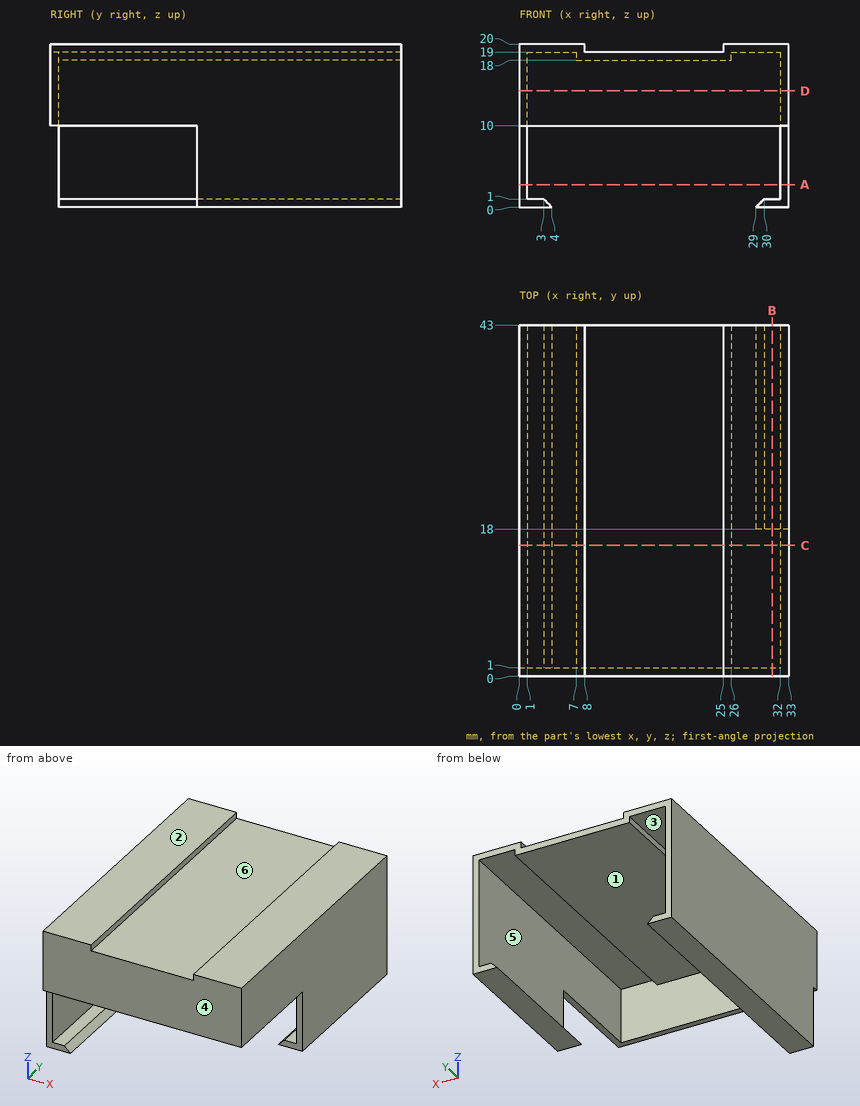
Print and shaded views of the part. All mm, measured from the part's lowest x, y and z. A direction names the side the tool comes from. Coordinates: 2 decimals unless noted, no trailing zeros. Order: outer loops, then holes, each group sorted by start corner. A loop starts at its lowest first (then second) coordinate and runs counter-clockwise, first axis right, second up. Notation, with made-up numbers: M 31,46.5 L 38,46.5 A9 cw 38,57.5 Z; hole C 20.25,22 d1. An arc over 180 degrees is marked long. Write each question's results on one line, items separated by ' | '. Start each with the question number.
Q1. Cut at C-C (y = 16). List the corners of the cut face in (x, z).
Q2. Which spindle directions (+Z, -Z, +X, -X, +Y, -Y) get a long thin tool onto all of the face, cutting with end or side? Do the marked faces 4, 5 and 6. Say none if no direction does.
Q3. Pull direction Z, two halves, no side cores. Call the marked faces 1, 2 and 3: +Z half, -Z half, draft (parallel to the pull), parting line (faces both ways), or undercut.
Q4. Cut at D-D (z = 14.25). List the corners of the cut face in (x, y).
Q5. Flat gauge pins, fed straight in: P1, Ø1.5, axis at x = 15, y = 29.5, coming from the +Z side; P2, Ø3, axis at x = 31.5, z = 7, coming from the -Y side; P3, Ø2.5, axis at x = 9, z = 14, coming from the +Y side. Where does each tip first touch, or does it go through?
Q6. Cut at A-A (z = 2.75). List the corners of the cut face in (x, y).
Q7. Cut at B-B (x = 31). List the corners of the cut face in (y, z), then the cut area to 3 significant figures.
Q8. Drill centre lines: probe 1 along X at (y, z) = (27, 15.5); probe 2 along Z at (x, y) = (2.5, 19); probe 3 along X at (y, z) = (4.5, 2.5). Where is each one in solid material? Low to high. Write a range as from..to.
Found:
1) outline: M 0,0 L 4,0 L 3,1 L 1,1 L 1,19 L 7,19 L 7,18 L 26,18 L 26,19 L 32,19 L 32,10 L 33,10 L 33,20 L 25,20 L 25,19 L 8,19 L 8,20 L 0,20 Z
2) face 4: +Z, -Z, +X, -X, -Y | face 5: +Y | face 6: +Z, +Y, -Y
3) face 1: -Z half | face 2: +Z half | face 3: undercut
4) outline: M 0,0 L 33,0 L 33,43 L 32,43 L 32,1 L 1,1 L 1,43 L 0,43 Z
5) P1: z = 19 | P2: y = 18 | P3: y = 1
6) outline: M 0,1 L 1,1 L 1,43 L 0,43 Z; M 32,18 L 33,18 L 33,43 L 32,43 Z
7) outline: M 0,10 L 1,10 L 1,19 L 43,19 L 43,20 L 0,20 Z; M 18,0 L 43,0 L 43,1 L 18,1 Z | area: 77.0 mm²
8) probe 1: 0..1, 32..33 | probe 2: 0..1, 19..20 | probe 3: 0..1
